Source: CAD feature listing. Evaluate the final solid. Frame: model axes, mm. A direction names the side the tool comes from. Give positions to 0.01 mm unless a question says otherwise; leave off trailing zeros. Write each loop counter-clockwise with the first axis right and the second up, starting at its lowest first coordinate (ties: lowest second). Pieces come first, ordered by that corner, then holes. Notation, with made-up numbers: (-26, 87) - (7, 87) arc R23 ccw to (7, 102) - close; hole circle Ø3 at (52, 83). An arc over 180 degrees is marked (long way). One line per question, with ' | ' between items. Start each with the question number.
(1) Section A-A, the plane y = 4.5. Return loops of the section in (x, z), plus the area to 3 significant figures.
(2) Draft query along Z for faces 4 (the flat face through (7.5, 1, 35)), 5 (the flat face through (0.7, -6.7, 1.5)), 6 (the flat face through (0, -7, 0)). Return one class per face: +Z half, -Z half, draft (parallel to the pull), parting line (faces both ways), or undercut.
(3) Access query for faces 1 (the flat face through (0.7, -6.7, 34.5)), 2 (the flat face through (0, -8.5, 18)), 3 (the flat face through (-7.5, 1, 1)). Directions: +Z, -Z, +X, -X, +Y, -Y. A direction counts if a zero-diameter tool reaches every point of the face in a straight line with its end or side. Return the directions, or none.
(4) Pin query (flat end, axial travel): pin 1 (1.5 mm diameter, centred on x = -1, z = 27, fed in from +Y); pin 2 (0.8 mm diameter, centred on x = -0.5, z = 34, fed in from +Y). Return the tip coordinate at first contact, or that it passes through.
(5) Ray query, line 1 (X direction, y = 1.5, z = 25.5); line 2 (Y direction, x = -2.75, z = 30.5). Return the intervals inside material, ascending. Write a range as [from, to].
(6) Section B-B, the plane z = 23.5. Return loops of the section in (x, y), plus the area to 3 significant figures.
(7) Section C-C, the plane x = 5. Return loops of the section in (y, z).
```python
from build123d import *

# Parameters (mm, degrees)
SKETCH1_W           = 19
SKETCH1_H           = 17
BOSS_EXTRUDE1_DEPTH = 36
SKETCH2_W           = 15
SKETCH2_H           = 36
CUT_EXTRUDE1_DEPTH  = 15
SKETCH3_W           = 19
SKETCH3_H           = 1.5
CUT_EXTRUDE2_DEPTH  = 15.5


with BuildPart() as part:
    # Sketch1 → Boss-Extrude1 (new body)
    with BuildSketch(Plane.XY):
        Rectangle(SKETCH1_W, SKETCH1_H)
    extrude(amount=BOSS_EXTRUDE1_DEPTH)

    # Sketch2 → Cut-Extrude1 (cut)
    with BuildSketch(Plane(origin=(0, 8.5, 0), x_dir=(1, 0, 0), z_dir=(0, 1, 0))):
        with Locations((0, -18)):
            Rectangle(SKETCH2_W, SKETCH2_H)
    extrude(amount=-CUT_EXTRUDE1_DEPTH, mode=Mode.SUBTRACT)

    # Sketch3 → Cut-Extrude2 (cut)
    with BuildSketch(Plane(origin=(0, 8.5, 0), x_dir=(1, 0, 0), z_dir=(0, 1, 0))):
        with Locations((0, -33.75)):
            Rectangle(SKETCH3_W, SKETCH3_H)
        with Locations((0, -2.25)):
            Rectangle(SKETCH3_W, SKETCH3_H)
    extrude(amount=-CUT_EXTRUDE2_DEPTH, mode=Mode.SUBTRACT)


solid = part.part
```
Check sheet entries:
1) outline: (-9.5, 0) - (-7.5, 0) - (-7.5, 1.5) - (-9.5, 1.5) - close; (-9.5, 3) - (-7.5, 3) - (-7.5, 33) - (-9.5, 33) - close; (-9.5, 34.5) - (-7.5, 34.5) - (-7.5, 36) - (-9.5, 36) - close; (7.5, 0) - (9.5, 0) - (9.5, 1.5) - (7.5, 1.5) - close; (7.5, 3) - (9.5, 3) - (9.5, 33) - (7.5, 33) - close; (7.5, 34.5) - (9.5, 34.5) - (9.5, 36) - (7.5, 36) - close | area: 132 mm²
2) face 4: draft | face 5: undercut | face 6: -Z half
3) face 1: +X, -X, +Y | face 2: +Z, -Z, +X, -X, -Y | face 3: +Z, -Z, +Y
4) pin 1: y = -6.5 | pin 2: y = -7
5) line 1: [-9.5, -7.5], [7.5, 9.5] | line 2: [-8.5, -6.5]
6) outline: (-9.5, -8.5) - (9.5, -8.5) - (9.5, 8.5) - (7.5, 8.5) - (7.5, -6.5) - (-7.5, -6.5) - (-7.5, 8.5) - (-9.5, 8.5) - close | area: 98.0 mm²
7) outline: (-8.5, 0) - (-6.5, 0) - (-6.5, 1.5) - (-7, 1.5) - (-7, 3) - (-6.5, 3) - (-6.5, 33) - (-7, 33) - (-7, 34.5) - (-6.5, 34.5) - (-6.5, 36) - (-8.5, 36) - close
